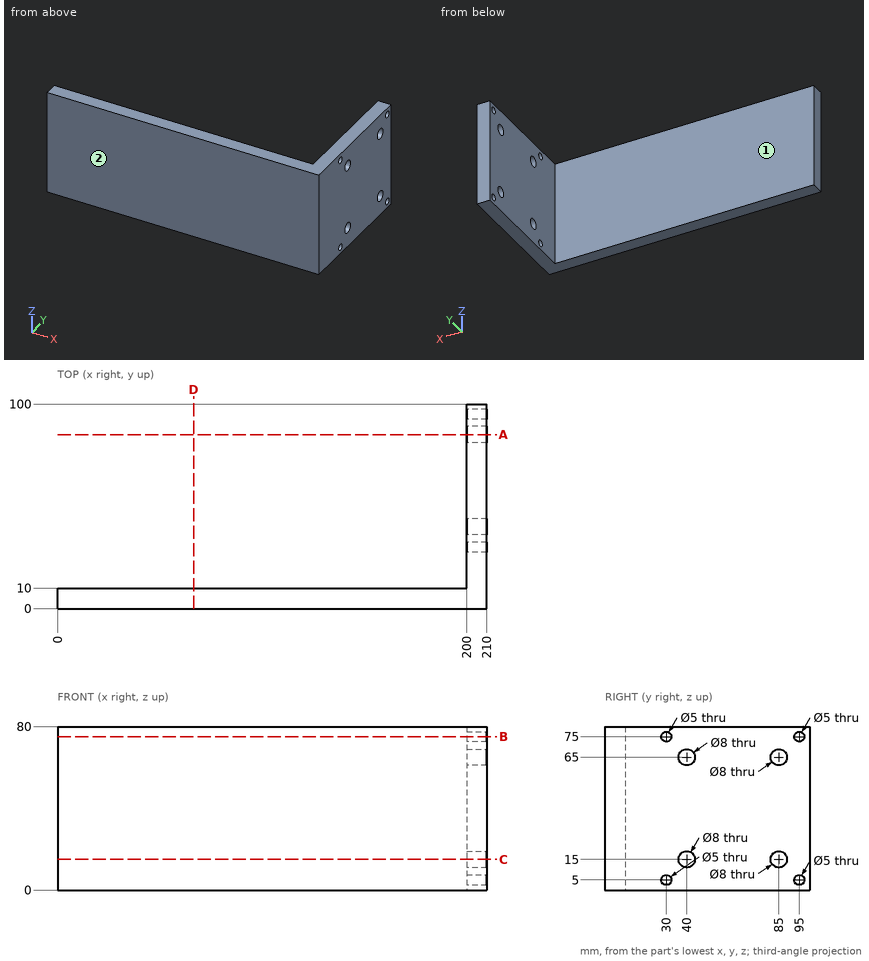
Check sheet for the drawn part. Datum: minimum x, y, z corner. Units: mm. A direction names the side the tool comes from. Round coordinates to 2 decimals unless told otherwise and drop trailing zeros. Order: outer loops, then holes, each group sorted by start corner. A loop starts at its lowest first (then second) coordinate and runs counter-clockwise, first axis right, second up.
(1) Cross-section at A-A, the plane y = 85. Enter the section's corners in (x, z), and give its area (3 significant figures).
(2) Access from +Z, -Z, +X, -X, +Y, -Y to the whole of each face (thin tool, end or side, straight path). Record for the marked faces 1 and 2.
(3) Cross-section at C-C, the plane z = 15. Enter the section's corners in (x, y), and give its area (3 significant figures).
(4) Cross-section at B-B, the plane z = 75. Enter the section's corners in (x, y), and give its area (3 significant figures).
(5) Scan lines: probe 1 along Y at (x, z) = (203, 15); probe 2 along Y at (x, z) = (141, 32); probe 3 along X at (y, z) = (61, 32). Record each from-to range of solid material in increasing order.
(6) Go/stop test with flat-tipped pins: P1, Ø13, axis at y = 85, z = 15, coming from the -X side; P2, Ø6, axis at x = 37.5, z = 19.5, coming from the +Y side. Record where each tip stops, or that it passes through.
(7) Cross-section at D-D, the plane x = 66.5. Enter the section's corners in (y, z), and give its area (3 significant figures).
Check sheet entries:
1. outline: (200, 0) - (210, 0) - (210, 11) - (200, 11) - close; (200, 19) - (210, 19) - (210, 61) - (200, 61) - close; (200, 69) - (210, 69) - (210, 80) - (200, 80) - close
1. area: 640 mm2
2. face 1: +Z, -Z, -X, +Y
2. face 2: +Z, -Z, +X, -X, -Y
3. outline: (0, 0) - (210, 0) - (210, 36) - (200, 36) - (200, 10) - (0, 10) - close; (200, 44) - (210, 44) - (210, 81) - (200, 81) - close; (200, 89) - (210, 89) - (210, 100) - (200, 100) - close
3. area: 2,840 mm2
4. outline: (0, 0) - (210, 0) - (210, 27.5) - (200, 27.5) - (200, 10) - (0, 10) - close; (200, 32.5) - (210, 32.5) - (210, 92.5) - (200, 92.5) - close; (200, 97.5) - (210, 97.5) - (210, 100) - (200, 100) - close
4. area: 2,900 mm2
5. probe 1: y = 0 to 36, 44 to 81, 89 to 100
5. probe 2: y = 0 to 10
5. probe 3: x = 200 to 210
6. P1: stops at x = 200
6. P2: stops at y = 10
7. outline: (0, 0) - (10, 0) - (10, 80) - (0, 80) - close
7. area: 800 mm2
